```python
from build123d import *

# Parameters (mm, degrees)
SKETCH3_R                = 43.942
BOSS_EXTRUDE1_DEPTH      = 15.24
BOSS_EXTRUDE2_REACH      = 2240.211
BOSS_EXTRUDE2_END_RADIUS = 78.322932
SKETCH4_W                = 3.175
SKETCH4_H                = 203.2
CUT_EXTRUDE1_REACH       = 2229.902
FILLET1_R                = 2.54
CIRPATTERN1_COUNT        = 4
FILLET1_OF_CIRPATTERN1_R = 2.54


with BuildPart() as part:
    # Sketch2 → Revolve1 (revolve)
    with BuildSketch(Plane(origin=(0, 0, 0), x_dir=(0, 0, -1), z_dir=(1, 0, 0))):
        with BuildLine():
            Line((161.200401562, 77.77155292), (2196.692901562, 77.77155292))
            Line((2196.692901562, 77.77155292), (2196.692901562, -0.55137908))
            Line((2196.692901562, -0.55137908), (4.482401562, -0.55137908))
            add(Edge.make_bspline(
                [(4.482401562, -0.55137908), (82.841401562, 77.77155292), (161.200401562, 77.77155292)],
                knots=[0.067653722, 0.067653722, 0.067653722, 0.915241247, 0.915241247, 0.915241247], degree=2))
        make_face()
    revolve(axis=Axis((0, -0.55137908, -2196.692901562), (0, 0, 1)))

    # Sketch3 → Boss-Extrude1 (add)
    with BuildSketch(Plane(origin=(0, 0, -2196.692901562), x_dir=(-1, 0, 0), z_dir=(0, 0, -1))):
        with Locations(Location((0, 0, 0), (0, 0, 270))):
            Circle(SKETCH3_R)
    extrude(amount=BOSS_EXTRUDE1_DEPTH)

    # Boss-Extrude2: up to this cylinder (the profile starts outside it)
    boss_extrude2_end = Plane(origin=(0, -0.55137908, -2091.917902), z_dir=(0, 0, -1)) * Cylinder(BOSS_EXTRUDE2_END_RADIUS, 4638.067864, mode=Mode.PRIVATE)
    # Sketch4 → Boss-Extrude2 (add, up to the surface)
    with BuildSketch(Plane(origin=(0, 254, 0), x_dir=(1, 0, 0), z_dir=(0, 1, 0)), mode=Mode.PRIVATE) as boss_extrude2_sk1:
        with Locations((0, 2091.917901562)):
            Rectangle(SKETCH4_W, SKETCH4_H)
    boss_extrude2_tool1 = extrude(boss_extrude2_sk1.sketch, amount=-BOSS_EXTRUDE2_REACH, mode=Mode.PRIVATE) - boss_extrude2_end
    boss_extrude2 = boss_extrude2_tool1.solids().sort_by_distance((0, 254, -2091.917902))[0]
    add(boss_extrude2)

    # Sketch5 → Cut-Extrude1 (cut, up to next)
    with BuildSketch(Plane.ZY.offset(1.5875), mode=Mode.PRIVATE) as cut_extrude1_sk1:
        Polygon((-2193.517901562, 223.805463028), (-2091.917901562, 223.805463028), (-1990.317901562, 77.755463028), (-1990.317901562, 254), (-2193.517901562, 254), align=None)
    cut_extrude1_tool1 = extrude(cut_extrude1_sk1.sketch, amount=-CUT_EXTRUDE1_REACH, mode=Mode.PRIVATE) & part.part
    cut_extrude1 = cut_extrude1_tool1.solids().sort_by_distance((-1.5875, 203.992033, -2054.843652))[0]
    add(cut_extrude1, mode=Mode.SUBTRACT)

    # Fillet1
    # the kernel refuses this fillet: 2.54 mm, written as the material it adds along each edge
    with BuildSketch(Plane(origin=(-1.5875, 77.755463028, -1984.191199419), x_dir=(-0.9993639751499004, -0.035660134220012574, 0), z_dir=(0, 0, -1))) as fillet1_piece_1_section:
        with BuildLine():
            CenterArc((2.450992889, 2.539698904), FILLET1_R, 182.043608468, 87.074170625)
            Line((-0.087391608, 2.449122163), (0, 0))
            ThreePointArc((0, 0), (1.205942189, 0.009284527), (2.411884379, 0))
        make_face()
    fillet1_piece_1 = extrude(amount=209.326702143, mode=Mode.PRIVATE)
    fillet1_piece_1 = split(fillet1_piece_1, bisect_by=Plane(origin=(-3.095055571, 77.697259455, -1990.27741212), z_dir=(0, -0.5710644881986003, -0.820905201785487)), keep=Keep.TOP, mode=Mode.PRIVATE)
    add(fillet1_piece_1)
    with BuildSketch(Plane(origin=(1.5875, 77.755463028, -1984.191199419), x_dir=(0.9993639751499004, -0.03566013422001344, 0), z_dir=(0, 0, -1))) as fillet1_piece_2_section:
        with BuildLine():
            CenterArc((2.450992889, -2.539698904), FILLET1_R, 90.882220907, 87.074170625)
            Line((-0.087391608, -2.449122163), (0, 0))
            ThreePointArc((0, 0), (1.205942189, -0.009284527), (2.411884379, 0))
        make_face()
    fillet1_piece_2 = extrude(amount=209.326702143, mode=Mode.PRIVATE)
    fillet1_piece_2 = split(fillet1_piece_2, bisect_by=Plane(origin=(3.095055571, 77.697259455, -1990.27741212), z_dir=(0, -0.5710644881986003, -0.820905201785487)), keep=Keep.TOP, mode=Mode.PRIVATE)
    add(fillet1_piece_2)

    # CirPattern1: Boss-Extrude2, Cut-Extrude1 ×4 about axis
    cirpattern1_axis = Axis((0, -0.55137908, 0), (0, 0, 1))
    add([boss_extrude2.rotate(cirpattern1_axis, i * 360 / CIRPATTERN1_COUNT) for i in range(1, CIRPATTERN1_COUNT)])
    add([cut_extrude1.rotate(cirpattern1_axis, i * 360 / CIRPATTERN1_COUNT) for i in range(1, CIRPATTERN1_COUNT)], mode=Mode.SUBTRACT)

    # Fillet1 of CirPattern1
    # the kernel refuses this fillet: 2.54 mm, written as the material it adds along each edge
    with BuildSketch(Plane(origin=(-78.306842107, -2.13887908, -1984.191199419), x_dir=(0.035660134220018555, -0.9993639751499002, 0), z_dir=(0, 0, -1))) as fillet1_of_cirpattern1_piece_1_section:
        with BuildLine():
            CenterArc((2.450992889, 2.539698904), FILLET1_OF_CIRPATTERN1_R, 182.043608468, 87.074170625)
            Line((-0.087391608, 2.449122163), (0, 0))
            ThreePointArc((0, 0), (1.205942189, 0.009284527), (2.411884379, 0))
        make_face()
    fillet1_of_cirpattern1_piece_1 = extrude(amount=209.326702143, mode=Mode.PRIVATE)
    fillet1_of_cirpattern1_piece_1 = split(fillet1_of_cirpattern1_piece_1, bisect_by=Plane(origin=(-78.248638535, -3.646434651, -1990.27741212), z_dir=(0.5710644881986003, 0, -0.820905201785487)), keep=Keep.TOP, mode=Mode.PRIVATE)
    add(fillet1_of_cirpattern1_piece_1)
    with BuildSketch(Plane(origin=(-78.306842107, 1.03612092, -1984.191199419), x_dir=(0.03566013422001241, 0.9993639751499004, 0), z_dir=(0, 0, -1))) as fillet1_of_cirpattern1_piece_2_section:
        with BuildLine():
            CenterArc((2.450992889, -2.539698904), FILLET1_OF_CIRPATTERN1_R, 90.882220907, 87.074170625)
            Line((-0.087391608, -2.449122163), (0, 0))
            ThreePointArc((0, 0), (1.205942189, -0.009284527), (2.411884379, 0))
        make_face()
    fillet1_of_cirpattern1_piece_2 = extrude(amount=209.326702143, mode=Mode.PRIVATE)
    fillet1_of_cirpattern1_piece_2 = split(fillet1_of_cirpattern1_piece_2, bisect_by=Plane(origin=(-78.248638535, 2.543676491, -1990.27741212), z_dir=(0.5710644881986003, 0, -0.820905201785487)), keep=Keep.TOP, mode=Mode.PRIVATE)
    add(fillet1_of_cirpattern1_piece_2)
    with BuildSketch(Plane(origin=(1.5875, -78.858221187, -1984.191199419), x_dir=(0.9993639751499, 0.035660134220024196, 0), z_dir=(0, 0, -1))) as fillet1_of_cirpattern1_piece_3_section:
        with BuildLine():
            CenterArc((2.450992889, 2.539698904), FILLET1_OF_CIRPATTERN1_R, 182.043608468, 87.074170625)
            Line((-0.087391608, 2.449122163), (0, 0))
            ThreePointArc((0, 0), (1.205942189, 0.009284527), (2.411884379, 0))
        make_face()
    fillet1_of_cirpattern1_piece_3 = extrude(amount=209.326702143, mode=Mode.PRIVATE)
    fillet1_of_cirpattern1_piece_3 = split(fillet1_of_cirpattern1_piece_3, bisect_by=Plane(origin=(3.095055571, -78.800017614, -1990.27741212), z_dir=(0, 0.5710644881986003, -0.820905201785487)), keep=Keep.TOP, mode=Mode.PRIVATE)
    add(fillet1_of_cirpattern1_piece_3)
    with BuildSketch(Plane(origin=(-1.5875, -78.858221187, -1984.191199419), x_dir=(-0.9993639751499004, 0.03566013422001241, 0), z_dir=(0, 0, -1))) as fillet1_of_cirpattern1_piece_4_section:
        with BuildLine():
            CenterArc((2.450992889, -2.539698904), FILLET1_OF_CIRPATTERN1_R, 90.882220907, 87.074170625)
            Line((-0.087391608, -2.449122163), (0, 0))
            ThreePointArc((0, 0), (1.205942189, -0.009284527), (2.411884379, 0))
        make_face()
    fillet1_of_cirpattern1_piece_4 = extrude(amount=209.326702143, mode=Mode.PRIVATE)
    fillet1_of_cirpattern1_piece_4 = split(fillet1_of_cirpattern1_piece_4, bisect_by=Plane(origin=(-3.095055571, -78.800017614, -1990.27741212), z_dir=(0, 0.5710644881986003, -0.820905201785487)), keep=Keep.TOP, mode=Mode.PRIVATE)
    add(fillet1_of_cirpattern1_piece_4)
    with BuildSketch(Plane(origin=(78.306842107, 1.03612092, -1984.191199419), x_dir=(-0.03566013422001241, 0.9993639751499004, 0), z_dir=(0, 0, -1))) as fillet1_of_cirpattern1_piece_5_section:
        with BuildLine():
            CenterArc((2.450992889, 2.539698904), FILLET1_OF_CIRPATTERN1_R, 182.043608468, 87.074170625)
            Line((-0.087391608, 2.449122163), (0, 0))
            ThreePointArc((0, 0), (1.205942189, 0.009284527), (2.411884379, 0))
        make_face()
    fillet1_of_cirpattern1_piece_5 = extrude(amount=209.326702143, mode=Mode.PRIVATE)
    fillet1_of_cirpattern1_piece_5 = split(fillet1_of_cirpattern1_piece_5, bisect_by=Plane(origin=(78.248638535, 2.543676491, -1990.27741212), z_dir=(-0.5710644881986003, 0, -0.820905201785487)), keep=Keep.TOP, mode=Mode.PRIVATE)
    add(fillet1_of_cirpattern1_piece_5)
    with BuildSketch(Plane(origin=(78.306842107, -2.13887908, -1984.191199419), x_dir=(-0.03566013422001242, -0.9993639751499004, 0), z_dir=(0, 0, -1))) as fillet1_of_cirpattern1_piece_6_section:
        with BuildLine():
            CenterArc((2.450992889, -2.539698904), FILLET1_OF_CIRPATTERN1_R, 90.882220907, 87.074170625)
            Line((-0.087391608, -2.449122163), (0, 0))
            ThreePointArc((0, 0), (1.205942189, -0.009284527), (2.411884379, 0))
        make_face()
    fillet1_of_cirpattern1_piece_6 = extrude(amount=209.326702143, mode=Mode.PRIVATE)
    fillet1_of_cirpattern1_piece_6 = split(fillet1_of_cirpattern1_piece_6, bisect_by=Plane(origin=(78.248638535, -3.646434651, -1990.27741212), z_dir=(-0.5710644881986003, 0, -0.820905201785487)), keep=Keep.TOP, mode=Mode.PRIVATE)
    add(fillet1_of_cirpattern1_piece_6)


solid = part.part
```
CAD build for the part. Positions are in the model's coordinates, mm. A direction names the side the tool comes from. Coordinates: 2 decimals unless noted, no trailing zeros. Write each loop counter-clockwise with the first axis right and the second up, starting at its lowest first coordinate (ties: lowest second). Pieces come first, ordered by that corner, then holes.
(1) 3-axis set-ups, long thin cutter, end or side, ignore diameter. For faces 1 (the face through (-13.199, -41.913, -2204.206)), 2 (the face through (-1.588, 153, -2114)), 3 (the face through (1.588, 153, -2114)): which of +Z, -Z, +X, -X, +Y, -Y reach the whole face in a straight line?
(2) Cut at C-C, the plane x = -109. List the corners of the cut face in (y, z).
(3) Drill centre lines: probe 1 along Y at (x, z) = (8, -1417); probe 2 along X at (y, z) = (-51, -1900); probe 3 along X at (y, z) = (-47.5, -108). Where is each one in solid material? Low to high.
(4) Flat gauge pins, fed straight in: pin 1 (4 mm diameter, centred on x = 1, y = -171, fed in from -Z); pin 2 (6 mm diameter, centred on x = -84, z = -998.5, fed in from +Y). Where does each tip first touch, or does it go through?
(5) Cut at B-B, the plane y = 122. List the corners of the cut face in (x, z), and give its area (3 significant figures).
(6) Cut at A-A, the plane z = -1187. List the corners of the cut face in (x, y).
Geometry says:
1. face 1: -Z
1. face 2: +Z, -Z, -X, +Y
1. face 3: +Z, -Z, +X, +Y
2. outline: (-2.14, -2193.52) - (1.04, -2193.52) - (1.04, -2011.67) - (-2.14, -2011.67) - close
3. probe 1: y = -78.46 to 77.36
3. probe 2: x = -59.91 to 59.91
3. probe 3: x = -50.97 to 50.97
4. pin 1: stops at z = -2193.52
4. pin 2: passes through
5. outline: (-1.59, -2193.52) - (1.59, -2193.52) - (1.59, -2021.1) - (-1.59, -2021.1) - close
5. area: 547 mm2
6. outline: circle Ø156.65 at (0, -0.55)
